from build123d import *

# Parameters (mm, degrees)
SKETCH1_W           = 180
SKETCH1_H           = 90
BOSS_EXTRUDE1_DEPTH = 5
SKETCH5_W           = 15.917599426
SKETCH5_H           = 22
SKETCH5_W_2         = 13.264666189
CUT_EXTRUDE3_DEPTH  = 101.747208398
SKETCH7_W           = 4
SKETCH7_H           = 22
CUT_EXTRUDE13_DEPTH = 101.747208398
SKETCH8_R           = 4
CUT_EXTRUDE14_DEPTH = 101.747208398
SKETCH9_W           = 45
SKETCH9_H           = 80
CUT_EXTRUDE15_DEPTH = 3
SKETCH10_W          = 46
SKETCH10_H          = 48
CUT_EXTRUDE16_DEPTH = 3


with BuildPart() as part:
    # Sketch1 → Boss-Extrude1 (new body)
    with BuildSketch(Plane.XY):
        Rectangle(SKETCH1_W, SKETCH1_H)
    extrude(amount=BOSS_EXTRUDE1_DEPTH)

    # Sketch5 → Cut-Extrude3 (cut, through all)
    with BuildSketch(Plane(origin=(0, 0, 0), x_dir=(-1, 0, 0), z_dir=(0, 0, -1))):
        with Locations((-82.041200287, 0)):
            Rectangle(SKETCH5_W, SKETCH5_H)
        with Locations((83.367666906, 0)):
            Rectangle(SKETCH5_W_2, SKETCH5_H)
    extrude(amount=-CUT_EXTRUDE3_DEPTH, mode=Mode.SUBTRACT)

    # Sketch7 → Cut-Extrude13 (cut, through all)
    with BuildSketch(Plane(origin=(0, 0, 0), x_dir=(-1, 0, 0), z_dir=(0, 0, -1))):
        with Locations((-72.082400574, 0)):
            Rectangle(SKETCH7_W, SKETCH7_H)
        with Locations((74.735333811, 0)):
            Rectangle(SKETCH7_W, SKETCH7_H)
    extrude(amount=-CUT_EXTRUDE13_DEPTH, mode=Mode.SUBTRACT)

    # Sketch8 → Cut-Extrude14 (cut, through all)
    with BuildSketch(Plane(origin=(0, 0, 0), x_dir=(-1, 0, 0), z_dir=(0, 0, -1))):
        with Locations((-81, 36)):
            Circle(SKETCH8_R)
        with Locations(Location((81, 36, 0), (0, 0, 180))):
            Circle(SKETCH8_R)
        with Locations((81, -36)):
            Circle(SKETCH8_R)
        with Locations(Location((-81, -36, 0), (0, 0, 180))):
            Circle(SKETCH8_R)
    extrude(amount=-CUT_EXTRUDE14_DEPTH, mode=Mode.SUBTRACT)

    # Sketch9 → Cut-Extrude15 (cut)
    with BuildSketch(Plane(origin=(0, 0, 0), x_dir=(-1, 0, 0), z_dir=(0, 0, -1))):
        with Locations((-27.5, 0)):
            Rectangle(SKETCH9_W, SKETCH9_H)
    extrude(amount=-CUT_EXTRUDE15_DEPTH, mode=Mode.SUBTRACT)

    # Sketch10 → Cut-Extrude16 (cut)
    with BuildSketch(Plane(origin=(0, 0, 0), x_dir=(-1, 0, 0), z_dir=(0, 0, -1))):
        with Locations((28, 0)):
            Rectangle(SKETCH10_W, SKETCH10_H)
    extrude(amount=-CUT_EXTRUDE16_DEPTH, mode=Mode.SUBTRACT)


solid = part.part
The listing builds one solid part. Answer for the finished solid, in the listing's coordinates (mm). A direction names the side the tool comes from. Coordinates: 2 decimals unless noted, no trailing zeros. Order: outer loops, then holes, each group sorted by start corner. A loop starts at its lowest first (then second) coordinate and runs counter-clockwise, first axis right, second up. Notation, with made-up numbers: (84, 42) -> (102, 42) arc R17 ccw to (102, 47) -> close; hole circle Ø7 at (65.5, -33.5). An arc over 180 degrees is marked (long way). Answer in a Markdown table with one row per item. Add a question column.
Item 1: Determine the mould class of faces 1 (the face through (90, -28, 2)), 2 (the face through (-81, -11, 2)), 3 (the face through (-1, -45, 2)) for opening direction Y: +Y half, -Y half, draft (parallel to the pull), parting line (faces both ways), or undercut.
Item 2: Find section D-D (y = 6.5). Write down the section's boundary in (x, z).
Item 3: Find section C-C (x = -81). Write down the section's boundary in (y, z).
Item 4: Find the intervals of material crossed by L1, parallel to Y at x = 81, z = 1.8; L2, parallel to Y at x = -42, z = 2.45; L3, parallel to X at y = -35.5, z = 1.25, in increasing order. Write a range as from..to.
Item 5: Find section B-B (z = 3.95). Write down the section's boundary in (x, y), then the cut area to 3 significant figures.
Item 6: Which of the six approach directions +Z, -Z, +X, -X, +Y, -Y give full straight-line access (tool end or side, diameter ignored) to faces 4 (the face through (80, -11, 2)), 5 (the face through (-28, 0, 3)), 6 (the face through (-72.735, 0, 2)), 7 (the face through (-1, 45, 2)), 8 (the face through (-81.521, 32.034, 2.465))?
Item 7: Find section A-A (y = -36). Write down the section's boundary in (x, z).
Item 8: Each of these flat-tipped pins is pushed along its axis until it touches: P1, Ø0.9, axis at y = -3.5, z = 1, coming from the +X side; P2, Ø6, axis at x = 25.5, y = -27.5, coming from the -Z side. Where does it stop, or does it pass through?
Result set:
| question | item | result |
|---|---|---|
| 1 | face 1 | draft |
| 1 | face 2 | undercut |
| 1 | face 3 | -Y half |
| 2 | outline | (-72.74, 0) -> (-51, 0) -> (-51, 3) -> (-5, 3) -> (-5, 0) -> (5, 0) -> (5, 3) -> (50, 3) -> (50, 0) -> (70.08, 0) -> (70.08, 5) -> (-72.74, 5) -> close |
| 3 | outline | (-45, 0) -> (-40, 0) -> (-40, 5) -> (-45, 5) -> close; (-32, 0) -> (-11, 0) -> (-11, 5) -> (-32, 5) -> close; (11, 0) -> (32, 0) -> (32, 5) -> (11, 5) -> close; (40, 0) -> (45, 0) -> (45, 5) -> (40, 5) -> close |
| 4 | L1 | y = -45..-40, -32..-11, 11..32, 40..45 |
| 4 | L2 | y = -45..-24, 24..45 |
| 4 | L3 | x = -90..-84.97, -77.03..5, 50..77.03, 84.97..90 |
| 5 | outline | (-90, -45) -> (90, -45) -> (90, -11) -> (70.08, -11) -> (70.08, 11) -> (90, 11) -> (90, 45) -> (-90, 45) -> (-90, 11) -> (-72.74, 11) -> (-72.74, -11) -> (-90, -11) -> close; hole circle Ø8 at (-81, -36); hole circle Ø8 at (-81, 36); hole circle Ø8 at (81, -36); hole circle Ø8 at (81, 36) |
| 5 | area | 15,200 mm² |
| 6 | face 4 | +Z, -Z, +X |
| 6 | face 5 | -Z |
| 6 | face 6 | +Z, -Z, -X |
| 6 | face 7 | +Z, -Z, +X, -X, +Y |
| 6 | face 8 | +Z, -Z |
| 7 | outline | (-90, 0) -> (-85, 0) -> (-85, 5) -> (-90, 5) -> close; (-77, 0) -> (5, 0) -> (5, 3) -> (50, 3) -> (50, 0) -> (77, 0) -> (77, 5) -> (-77, 5) -> close; (85, 0) -> (90, 0) -> (90, 5) -> (85, 5) -> close |
| 8 | P1 | stops at x = 70.08 |
| 8 | P2 | stops at z = 3 |
